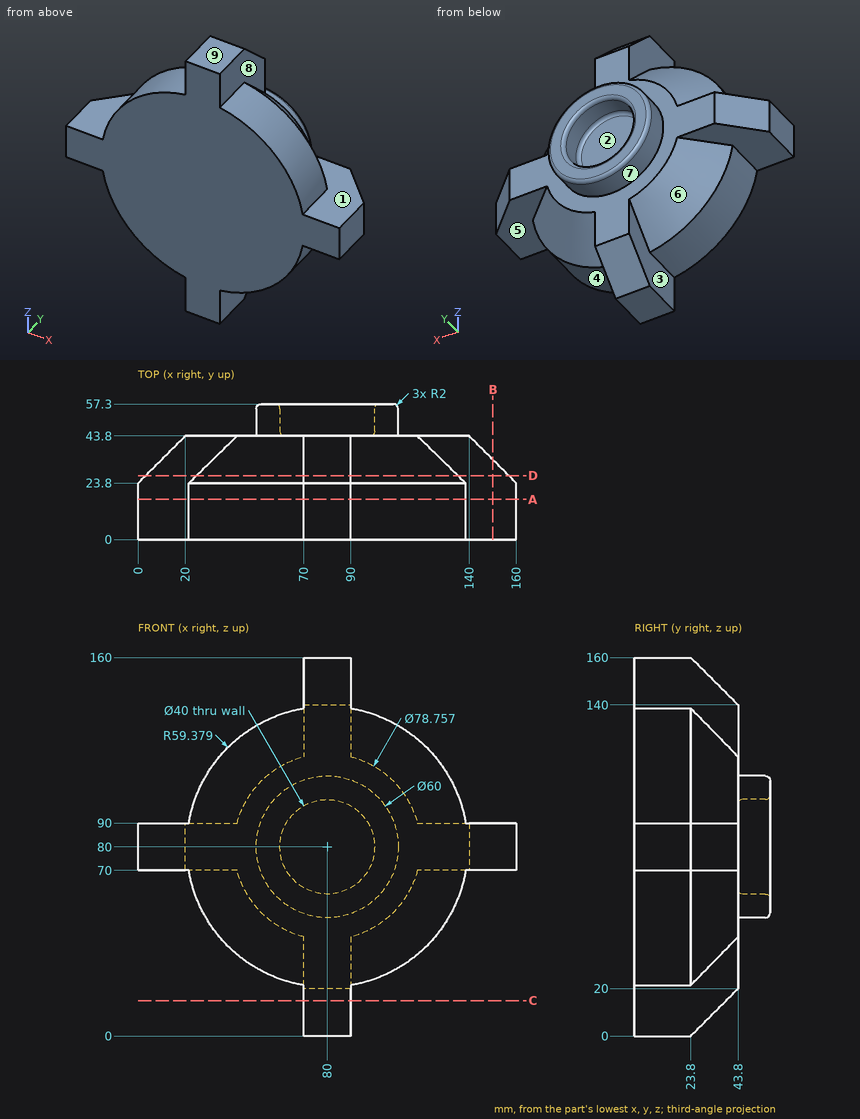
Answer from the drawing. Dimensions are ordinates in mm from the lowest x, y and z of the part. A direction names the side the tool comes from. Give positions to 0.01 mm unless a question says otherwise; leave off trailing zeros. Loops run counter-clockwise (first coordinate to the right, second up) from the corner with the lowest first, then second, coordinate; pieces in that order, holes last. Notation, with made-up numbers: M 14,41 L 34,41 A17 ccw 34,50 Z; hole C 48.5,21.25 d6. An arc over 180 degrees is marked long. One line per item, written item: value.
Q1. For the marked faces 5, 6, 7, 8 and 9, determine the directions among +Z, -Z, +X, -X, +Y, -Y from which every point of the face is accessible in a straight line to the end or side of a thin tool.
Working result:
face 5: -Z, +X, +Y
face 6: -Z, -X, +Y
face 7: +Y
face 8: +Z, +X, +Y
face 9: +Z, +X, -X, +Y, -Y
Q2. A cutting plane is placed at C-C on z = 15. Determine the outline of the cut face in (x, y), then the cut area to 3 significant figures.
Working result:
outline: M 70,0 L 90,0 L 90,38.8 L 70,38.8 Z
area: 776 mm^2
Q3. A cutting plane is placed at A-A on y = 17. Determine the outline of the cut face in (x, z).
Working result:
outline: M 0,70 L 21.47,70 A59.38 ccw 70,21.47 L 70,0 L 90,0 L 90,21.47 A59.38 ccw 138.53,70 L 160,70 L 160,90 L 138.53,90 A59.38 ccw 90,138.53 L 90,160 L 70,160 L 70,138.53 A59.38 ccw 21.47,90 L 0,90 Z
Q4. A cutting plane is placed at B-B on x = 150. Determine the outline of the cut face in (y, z).
Working result:
outline: M 0,70 L 33.8,70 L 33.8,90 L 0,90 Z
Q5. Find the intervals of material crossed by line 1 (Z direction, x = 80, y = 52.25); line 2 (Y direction, x = 137, z = 85); line 3 (X direction, y = 29, z = 12), in increasing order. Write a range as from..to.
Working result:
line 1: z = 50..60, 100..110
line 2: y = 0..43.8
line 3: x = 70..90
Q6. Determine the mould class of the marked faces 1, 2, 3 and 4 for opening direction Z: +Z half, -Z half, draft (parallel to the pull), parting line (faces both ways), or undercut.
Working result:
face 1: +Z half
face 2: undercut
face 3: draft
face 4: -Z half
Q7. A cutting plane is placed at D-D on y = 27. Determine the outline of the cut face in (x, z).
Working result:
outline: M 3.2,70 L 24.72,70 A56.18 ccw 70,24.72 L 70,3.2 L 90,3.2 L 90,24.72 A56.18 ccw 135.28,70 L 156.8,70 L 156.8,90 L 135.28,90 A56.18 ccw 90,135.28 L 90,156.8 L 70,156.8 L 70,135.28 A56.18 ccw 24.72,90 L 3.2,90 Z
Q8. Flat-ended cylindrical pins translate along their axes: P1, Ø1, axis at y = 36, z = 119.5, coming from the -X side (1 decimal); P2, Ø1, axis at y = 41.5, z = 29, coming from the -X side; P3, Ø3, axis at x = 82.5, y = 45, coming from the +Z side. Find the tip coordinate at first contact, or state that the pin passes through.
Working result:
P1: stops at x = 53
P2: stops at x = 70
P3: stops at z = 140.3
